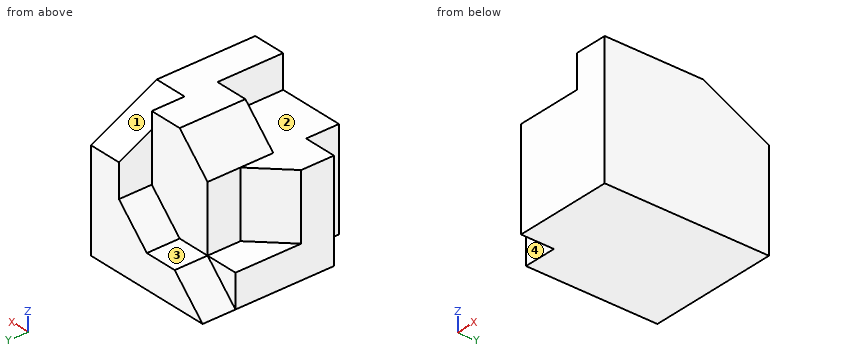
from build123d import *

# Parameters (mm, degrees)
SKETCH1_W           = 40
SKETCH1_H           = 40
BOSS_EXTRUDE1_DEPTH = 50
CUT_EXTRUDE1_DEPTH  = 10
CUT_EXTRUDE2_DEPTH  = 10
CUT_EXTRUDE5_DEPTH  = 10
CUT_EXTRUDE6_DEPTH  = 30
CUT_EXTRUDE7_DEPTH  = 10
SKETCH10_W          = 10
SKETCH10_H          = 10
CUT_EXTRUDE8_DEPTH  = 10
SKETCH11_W          = 30
SKETCH11_H          = 20
CUT_EXTRUDE9_DEPTH  = 10
SKETCH13_W          = 10
SKETCH13_H          = 10
CUT_EXTRUDE10_DEPTH = 31


with BuildPart() as part:
    # Sketch1 → Boss-Extrude1 (new body)
    with BuildSketch(Plane(origin=(0, 0, 0), x_dir=(1, 0, 0), z_dir=(0, 1, 0))):
        Rectangle(SKETCH1_W, SKETCH1_H)
    extrude(amount=BOSS_EXTRUDE1_DEPTH)

    # Sketch2 → Cut-Extrude1 (cut)
    with BuildSketch(Plane(origin=(0, 50, 0), x_dir=(1, 0, 0), z_dir=(0, 1, 0))):
        Polygon((-20, 20), (-10, 10), (0, 10), (10, 0), (10, -20), (-20, -20), align=None)
    extrude(amount=-CUT_EXTRUDE1_DEPTH, mode=Mode.SUBTRACT)

    # Sketch3 → Cut-Extrude2 (cut)
    with BuildSketch(Plane(origin=(20, 0, 0), x_dir=(0, 0, -1), z_dir=(1, 0, 0))):
        Polygon((-20, 50), (-10, 50), (-20, 30), align=None)
    extrude(amount=-CUT_EXTRUDE2_DEPTH, mode=Mode.SUBTRACT)

    # Sketch7 → Cut-Extrude5 (cut)
    with BuildSketch(Plane(origin=(0, 40, 0), x_dir=(1, 0, 0), z_dir=(0, 1, 0))):
        Polygon((0, -20), (-10, -10), (-10, 10), (-20, 10), (-20, -20), align=None)
    extrude(amount=-CUT_EXTRUDE5_DEPTH, mode=Mode.SUBTRACT)

    # Sketch8 → Cut-Extrude6 (cut)
    with BuildSketch(Plane.XY.offset(20)):
        Polygon((-10, 30), (-20, 20), (-20, 30), align=None)
    extrude(amount=-CUT_EXTRUDE6_DEPTH, mode=Mode.SUBTRACT)

    # Sketch9 → Cut-Extrude7 (cut)
    with BuildSketch(Plane(origin=(0, 30, 0), x_dir=(1, 0, 0), z_dir=(0, 1, 0))):
        Polygon((0, -20), (-10, -10), (-10, -20), align=None)
    extrude(amount=-CUT_EXTRUDE7_DEPTH, mode=Mode.SUBTRACT)

    # Sketch10 → Cut-Extrude8 (cut)
    with BuildSketch(Plane(origin=(-10, 0, 0), x_dir=(0, 0, -1), z_dir=(1, 0, 0))):
        with Locations((-15, 25)):
            Rectangle(SKETCH10_W, SKETCH10_H)
    extrude(amount=-CUT_EXTRUDE8_DEPTH, mode=Mode.SUBTRACT)

    # Sketch11 → Cut-Extrude9 (cut)
    with BuildSketch(Plane.XY.offset(20)):
        with Locations((-5, 10)):
            Rectangle(SKETCH11_W, SKETCH11_H)
    extrude(amount=-CUT_EXTRUDE9_DEPTH, mode=Mode.SUBTRACT)

    # Sketch13 → Cut-Extrude10 (cut, through all)
    with BuildSketch(Plane.XY.offset(10)):
        with Locations((-15, 5)):
            Rectangle(SKETCH13_W, SKETCH13_H)
    extrude(amount=-CUT_EXTRUDE10_DEPTH, mode=Mode.SUBTRACT)


solid = part.part
Part model, mm, in its own coordinate system. Face numbers are marked on the shaded views. A direction names the side the tool comes from. Round coordinates to 2 decimals unless told otherwise and drop trailing zeros. Write each loop counter-clockwise with the first axis right and the second up, starting at its lowest first coordinate (ties: lowest second). Pieces come first, ordered by that corner, then holes. Notation, with made-up numbers: (54, -24) - (109, -24) arc R19 cw to (109, -11) - close; hole circle Ø9 at (-10, 22.25). An arc over 180 degrees is marked (long way). Use CSV: the item, a comma, the result in double quotes.
Item 1: Wall check: L1, parallel to X at y = 8, z = -8.5; L2, parallel to Y at x = 0.5, z = -6.5; L3, parallel to Z at x = -1.5, y = 47.5. Give the ranges that are in metal, low to high.
Results list:
L1,"x = -10 to 20"
L2,"y = 0 to 40"
L3,"z = -20 to -10"
Item 2: Slice it at B-B, the plane z = 11. Write the cut outline in (x, y), then the cut area to 3 significant figures.
Results list:
outline,"(-9, 20) - (10, 20) - (10, 0) - (20, 0) - (20, 48) - (10, 48) - (10, 40) - (-9, 40) - close"
area,"860 mm²"
Item 3: Slice it at A-A, the plane y = 34. Write the cut outline in (x, z).
Results list:
outline,"(-20, -20) - (20, -20) - (20, 18) - (10, 18) - (10, 20) - (0, 20) - (-10, 10) - (-10, -10) - (-20, -10) - close"
Item 4: Slice it at D-D, the plane z = -6. Write the cut outline in (x, y).
Results list:
outline,"(-20, 10) - (-10, 10) - (-10, 0) - (20, 0) - (20, 50) - (4, 50) - (4, 40) - (-10, 40) - (-10, 30) - (-20, 20) - close"
Item 5: Flat gauge pins, fed straight in: P1, Ø11, axis at x = -16.5, z = -7.5, coming from the -Y side; P2, Ø2, axis at x = -15.5, y = 20.5, coming from the +Z side; P3, Ø8, axis at y = 47, z = 4.5, coming from the -X side. Where does each tip first touch, or does it go through?
Results list:
P1,"stops at y = 10"
P2,"stops at z = 10"
P3,"stops at x = 10"
Item 6: Slice it at C-C, the plane x = -15. Write the cut outline in (y, z), then the cut area to 3 significant figures.
Results list:
outline,"(10, -20) - (50, -20) - (50, -15) - (40, -15) - (40, -10) - (25, -10) - (25, 10) - (10, 10) - close"
area,"650 mm²"
Item 7: Tool access for the marked faces 1, 2, 3 and 4: list every direction of +Z, -Z, +X, -X, +Y, -Y with a clear straight run to the whole face (end or side of a thin tool).
Results list:
face 1,"+Z, +X, +Y"
face 2,"+Z, -X, -Y"
face 3,"+Z, -X, +Y"
face 4,"+Z, -Z, -X, -Y"
